Here's how the part is built. I have some questions about the finished solid (model axes, mm). Face numbers are marked on the shaded views. A direction names the side the tool comes from. Round coordinates to 2 decimals unless told otherwise and drop trailing zeros. Loops run counter-clockwise (first coordinate to the right, second up) from the corner with the lowest first, then second, coordinate; pieces in that order, holes last. Notation, with made-up numbers: (-5.75, 52.25) -> (7.25, 52.25) arc R16 ccw to (7.25, 64.25) -> close; hole circle Ø1 at (-3.75, -26.5). An arc over 180 degrees is marked (long way). Use one line per item in the form item = value. Start each with the question number.
Item 1: If we section it at C-C (x = -1.75): Write out the boundary of the cut face in (y, z), then the cut area to 3 significant figures.
Item 2: Thinking about a two-plate mould opening in Z: for the marked faces 3, 4 and 5, which applies, released by +Z, released by -Z, zero draft, split by the parting line, or undercut?
Item 3: I'm going to push flat-ended pins straight in: pin 1 Ø3.5 at (y, z) = (5.08, -1.48) entering from -X; pin 2 Ø4 at (x, z) = (-5.5, 1) entering from +Y. Where does each tip first touch, or does it pass through?
Item 4: If we section it at B-B (z = -1.75): Write out the boundary of the cut face in (x, y), then the cut area to 3 significant figures.
Item 5: For the marked faces 1 and 2, which set-ups out of +Z, -Z, +X, -X, +Y, -Y let a thin tool reach every point of the face, with its end or its side?
Item 6: If we section it at D-D (z = 1.5): Write out the boundary of the cut face in (x, y).
Item 7: If I drill on L1, parallel to Z at x = -0.75, y = 1; L2, parallel to X at y = 7, z = -6.5; L3, parallel to Y at x = 0.75, z = -5.75, over which ranges is the centre line in solid material (lowest first)? Write a range as [from, to].
Item 8: If we section it at A-A (y = 5.08): Write out the boundary of the cut face in (x, z).
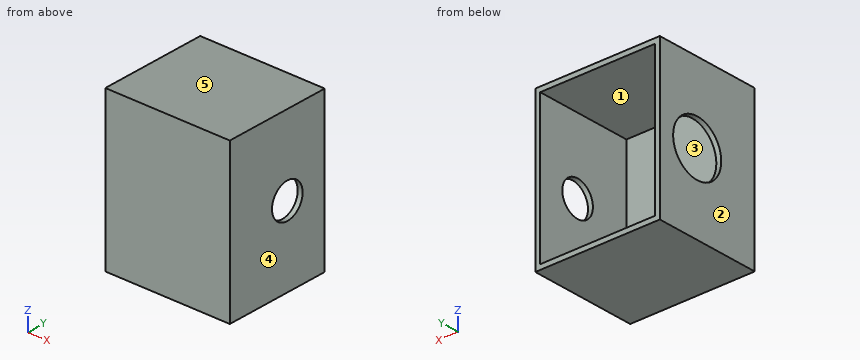
```python
from build123d import *

# Parameters (mm, degrees)
SKETCH1_W                 = 9.652
SKETCH1_H                 = 12.192
BOSS_EXTRUDE1_DEPTH       = 8.382
SKETCH4_W                 = 8.89
SKETCH4_H                 = 11.43
CUT_EXTRUDE1_DEPTH        = 7.62
CUT_EXTRUDE2_REACH        = 11.652
SKETCH6_R                 = 2.12471
F_6_32_TAPPED_HOLE2_D     = 2.7051
F_6_32_TAPPED_HOLE2_DEPTH = 0.381


with BuildPart() as part:
    # Sketch1 → Boss-Extrude1 (new body)
    with BuildSketch(Plane(origin=(0, 0, 0), x_dir=(1, 0, 0), z_dir=(0, 1, 0))):
        with Locations((-3.14180083, 1.47973444)):
            Rectangle(SKETCH1_W, SKETCH1_H)
    extrude(amount=BOSS_EXTRUDE1_DEPTH)

    # Sketch4 → Cut-Extrude1 (cut)
    with BuildSketch(Plane(origin=(0, 8.382, 0), x_dir=(1, 0, 0), z_dir=(0, 1, 0))):
        with Locations((-3.14180083, 1.47973444)):
            Rectangle(SKETCH4_W, SKETCH4_H)
    extrude(amount=-CUT_EXTRUDE1_DEPTH, mode=Mode.SUBTRACT)

    # Sketch6 → Cut-Extrude2 (cut, up to next)
    with BuildSketch(Plane.ZY.offset(7.96780083), mode=Mode.PRIVATE) as cut_extrude2_sk1:
        with Locations((-1.47973444, 5.08)):
            Circle(SKETCH6_R)
    cut_extrude2_tool1 = extrude(cut_extrude2_sk1.sketch, amount=-CUT_EXTRUDE2_REACH, mode=Mode.PRIVATE) & part.part
    add(cut_extrude2_tool1.solids().sort_by_distance((-7.967801, 5.08, -1.479734))[0], mode=Mode.SUBTRACT)

    # #6-32 Tapped Hole2
    with Locations(Plane(origin=(1.68419917, 0, 0), x_dir=(0, 0, -1), z_dir=(1, 0, 0))):
        with Locations((1.47973444, 5.08)):
            Hole(F_6_32_TAPPED_HOLE2_D / 2, depth=F_6_32_TAPPED_HOLE2_DEPTH)


solid = part.part
```
Values found:
q1.outline = (0, -7.58) -> (8.38, -7.58) -> (8.38, -7.19) -> (0.76, -7.19) -> (0.76, 4.24) -> (8.38, 4.24) -> (8.38, 4.62) -> (0, 4.62) -> close
q1.area = 15.1 mm2
q2.face_3 = undercut
q2.face_4 = zero draft
q2.face_5 = released by +Z
q3.pin_1 = 1.3
q3.pin_2 = 0.76
q4.outline = (-7.97, 0) -> (1.68, 0) -> (1.68, 3.75) -> (1.3, 3.75) -> (1.3, 0.76) -> (-7.59, 0.76) -> (-7.59, 2.97) -> (-7.97, 2.97) -> close; (-7.97, 7.19) -> (-7.59, 7.19) -> (-7.59, 8.38) -> (-7.97, 8.38) -> close; (1.3, 6.41) -> (1.68, 6.41) -> (1.68, 8.38) -> (1.3, 8.38) -> close
q4.area = 10.5 mm2
q5.face_1 = +Y
q5.face_2 = +Z, -Z, -X, +Y, -Y
q6.outline = (-7.97, 0) -> (1.68, 0) -> (1.68, 8.38) -> (1.3, 8.38) -> (1.3, 0.76) -> (-7.59, 0.76) -> (-7.59, 8.38) -> (-7.97, 8.38) -> close
q7.L1 = [-7.58, -7.19], [4.24, 4.62]
q7.L2 = [-7.97, -7.59], [1.3, 1.68]
q7.L3 = [0, 0.76]
q8.outline = (-7.97, -7.58) -> (1.68, -7.58) -> (1.68, -2.83) -> (1.3, -2.83) -> (1.3, -7.19) -> (-7.59, -7.19) -> (-7.59, -3.6) -> (-7.97, -3.6) -> close; (-7.97, 0.64) -> (-7.59, 0.64) -> (-7.59, 4.24) -> (1.3, 4.24) -> (1.3, -0.13) -> (1.68, -0.13) -> (1.68, 4.62) -> (-7.97, 4.62) -> close
